CAD build for the part. Positions are in the model's coordinates, mm. A direction names the side the tool comes from. Give positions to 0.01 mm unless a question says otherwise; leave off trailing zeros. Write each loop counter-clockwise with the first axis right and the second up, starting at its lowest first coordinate (ties: lowest second). Pieces come first, ordered by that corner, then holes. Notation, with made-up numbers: (17.25, 40) - (60.25, 40) arc R18 ccw to (60.25, 48) - close; hole circle Ø5 at (40, 80.5). An arc over 180 degrees is marked (long way). Put each result on its own line as item: value. Start each with the question number.
1. Mould opens along X. For faces 4 (the flat face through (15.6, -4, 0)), 5 (the cylindrical face through (8.619, -2.126, -5.127)), 6 (the cylindrical face through (-1.514, -10.108, 0.477)) say: +X half, -X half, draft (parallel to the pull), parting line (faces both ways), or undercut.
2. Cut at B-B on y = -14. List the corners of the cut face in (x, z) (1 decimal), and give its area (3 significant figures).
3. Wall check: line 1 (Y direction, x = 8.75, z = 0) (3 decimals); line 2 (Y direction, x = 5.75, z = 0) (3 decimals); line 3 (Y direction, x = -2, z = 3.5). Give the ranges that are in metal, low to high.
4. Tool access for faces 1 (the conical face through (2.87, -7.92, 5)), 2 (the conical face through (2.892, -7.918, -4.981)), 3 (the conical face through (5.76, -7.92, 0.01)): list every direction of +Z, -Z, +X, -X, +Y, -Y with a clear straight run to the whole face (end or side of a thin tool).
5. Drop flat-ended pins along their axis: pin 1 (5.5 mm diameter, centred on x = 2.5, z = 1.5, fed in from +Y); pin 2 (1 mm diameter, centred on x = 13.5, z = 1, fed in from -Y); pin 3 (2.5 mm diameter, centred on x = 0, z = 0, fed in from +Y); pin 4 (1 mm diameter, centred on x = 0.5, y = -15, fed in from -Z). Give the stop position or say it passes through.
6. Cut at A-A on y = -9. List the corners of the cut face in (x, z) (1 decimal), and give its area (3 significant figures).
from build123d import *

# Parameters (mm, degrees)
SKETCH1_R             = 4
BASE_EXTRUDE_DEPTH    = 3.6
RBODY_SKETCH_R        = 5.55
RBODY_DEPTH           = 9.6
ELBOW_ANGLE           = 90
SKETCH3_R             = 4
BOSS_EXTRUDE1_DEPTH   = 7.8
NUT_DEPTH             = 2.8
RTUBE_START           = -13.3
RTUBE_SKETCH_R        = 3.175
RTUBE_DEPTH           = 13.3
RTUBE_RADIUS_R        = 0.5
DIAMETER_R            = 1.5875
SKETCH4_W             = 3.5
SKETCH4_H             = 3.95
PORT_THREADS_REACH    = 30.544
PORT_THREADS_SKETCH_R = 1.5875


with BuildPart() as part:
    # Sketch1 → Base-Extrude (new body)
    with BuildSketch(Plane(origin=(0, 0, 0), x_dir=(0, 0, -1), z_dir=(1, 0, 0))):
        with Locations(Location((0, 0, 0), (0, 0, 180))):
            Circle(SKETCH1_R)
    extrude(amount=BASE_EXTRUDE_DEPTH)

    # RBody_Sketch → RBody (add)
    with BuildSketch(Plane(origin=(3.6, 0, 0), x_dir=(0, 0, -1), z_dir=(1, 0, 0))):
        Circle(RBODY_SKETCH_R)
    extrude(amount=RBODY_DEPTH)

    # RBody_Chamfer: read off the stored shape, not the designer's step
    # RBody_Chamfer outline → RBody_Chamfer (revolve, cut)
    with BuildSketch(Plane.YX):
        Polygon((5.55, 4.164153863), (4, 3.6), (5.55, 3.6), align=None)
    revolve(axis=Axis((0, 0, 0), (1, 0, 0)), mode=Mode.SUBTRACT)

    # RRelease_Sketch → RRelease (revolve)
    with BuildSketch(Plane.XY, mode=Mode.PRIVATE) as rrelease_sk:
        with BuildLine():
            Line((13.2, 3.925), (14.1, 3.925))
            Line((14.1, 3.925), (14.1, 5.025))
            Line((14.1, 5.025), (15.1, 5.025))
            ThreePointArc((15.1, 5.025), (15.453553391, 4.878553391), (15.6, 4.525))
            Line((15.6, 4.525), (15.6, 0))
            Line((15.6, 0), (13.2, 0))
            Line((13.2, 0), (13.2, 3.925))
        make_face()
    revolve(rrelease_sk.sketch.rotate(Axis((12.597722381, 0, 0), (1, 0, 0)), 90), axis=Axis((12.597722381, 0, 0), (1, 0, 0)))

    # Elbow_Sketch → Elbow (revolve)
    with BuildSketch(Plane.ZY):
        with BuildLine():
            Line((-4, 0), (4, 0))
            ThreePointArc((4, 0), (0, 4), (-4, 0))
        make_face()
    revolve(axis=Axis((0, 0, -6.487672297), (0, 0, 1)), revolution_arc=ELBOW_ANGLE)

    # Sketch3 → Boss-Extrude1 (add)
    with BuildSketch(Plane.XZ):
        with Locations(Location((0, 0, 0), (0, 0, 90))):
            Circle(SKETCH3_R)
    extrude(amount=BOSS_EXTRUDE1_DEPTH)

    # Nut_Sketch → Nut (add)
    with BuildSketch(Plane(origin=(0, -10.6, 0), x_dir=(-1, 0, 0), z_dir=(0, 1, 0))):
        Polygon((6.414361491, 0), (3.207180745, 5.555), (-3.207180745, 5.555), (-6.414361491, 0), (-3.207180745, -5.555), (3.207180745, -5.555), align=None)
    extrude(amount=NUT_DEPTH)

    # Nut_Chamfer_Sketch → Nut_Chamfer (revolve, cut)
    with BuildSketch(Plane.XY):
        Polygon((-5.555, -7.8), (-6.414361491, -7.8), (-6.414361491, -8.296152588), align=None)
        Polygon((-6.414361491, -10.103847412), (-5.555, -10.6), (-6.414361491, -10.6), align=None)
    revolve(axis=Axis((0, -1.551633987, 0), (0, 1, 0)), mode=Mode.SUBTRACT)

    # Threads_Sketch → Threads (revolve)
    with BuildSketch(Plane.XY):
        Polygon((-5.247489296, -10.6), (-5.026347442, -17.7), (0, -17.7), (0, -10.6), align=None)
    revolve(axis=Axis((0, 0, 0), (0, -1, 0)))

    # Thread_Chamfer: read off the stored shape, not the designer's step
    # Thread_Chamfer outline → Thread_Chamfer (revolve, cut)
    with BuildSketch(Plane.XY):
        Polygon((5.034384454, -17.441962988), (4.776347442, -17.7), (5.034384454, -17.7), align=None)
    revolve(axis=Axis((0, 0, 0), (0, 1, 0)), mode=Mode.SUBTRACT)

    # RTube_Sketch → RTube (cut)
    with BuildSketch(Plane(origin=(15.6, 0, 0), x_dir=(0, 0, -1), z_dir=(1, 0, 0)).offset(RTUBE_START)):
        Circle(RTUBE_SKETCH_R)
    extrude(amount=RTUBE_DEPTH, mode=Mode.SUBTRACT)

    # RTube_Radius
    rtube_radius_edges = [part.edges().sort_by_distance(p)[0] for p in [
        (15.6, 0, 3.175),
    ]]
    fillet(rtube_radius_edges, radius=RTUBE_RADIUS_R)

    # Port_Curve: sweep along a path in Profile
    with BuildLine(Plane.XY) as port_curve_path:
        ThreePointArc((2.3, 0), (0.673654403, -0.673654403), (0, -2.3))
    # Diameter → Port_Curve (sweep, cut)
    with BuildSketch(Plane(origin=(2.3, 0, 0), x_dir=(0, 0, -1), z_dir=(1, 0, 0))):
        Circle(DIAMETER_R)
    sweep(path=port_curve_path.line, mode=Mode.SUBTRACT)

    # Sketch4 → Revolve1 (revolve)
    with BuildSketch(Plane.XY):
        with Locations((-1.75, -12.575)):
            Rectangle(SKETCH4_W, SKETCH4_H)
    revolve(axis=Axis((0, 0, 0), (0, -1, 0)))

    # Port_Threads_Sketch → Port_Threads (cut, up to next)
    with BuildSketch(Plane(origin=(0, -17.7, 0), x_dir=(-1, 0, 0), z_dir=(0, 1, 0)), mode=Mode.PRIVATE) as port_threads_sk1:
        Circle(PORT_THREADS_SKETCH_R)
    port_threads_tool1 = extrude(port_threads_sk1.sketch, amount=PORT_THREADS_REACH, mode=Mode.PRIVATE) & part.part
    add(port_threads_tool1.solids().sort_by_distance((0, -17.7, 0))[0], mode=Mode.SUBTRACT)


solid = part.part
Report:
1. face 4: +X half
1. face 5: draft
1. face 6: undercut
2. outline: circle Ø10.3 at (0, 0); hole circle Ø3.2 at (0, 0)
2. area: 75.1 mm²
3. line 1: y = -5.55 to -3.175, 3.175 to 5.55
3. line 2: y = -10.487 to -7.913, -5.55 to -3.175, 3.175 to 5.55
3. line 3: y = -17.7 to -7.8
4. face 1: +Z, +X
4. face 2: -Z, +X
4. face 3: +X
5. pin 1: stops at y = 5.55
5. pin 2: stops at y = -5.52
5. pin 3: stops at y = 4
5. pin 4: stops at z = -5.12
6. outline: (-6.4, 0) - (-3.2, -5.6) - (3.2, -5.6) - (6.4, 0) - (3.2, 5.6) - (-3.2, 5.6) - close; hole circle Ø3.2 at (0, 0)
6. area: 99.0 mm²
